```python
from build123d import *

# Parameters (mm, degrees)
SKETCH1_W              = 150
SKETCH1_H              = 150
BOSS_EXTRUDE1_DEPTH    = 25
SKETCH2_R              = 30
BOSS_EXTRUDE2_DEPTH    = 9
CHAMFER1_SIZE          = 2
M25X1_5_TAPPED_HOLE1_D = 23.5
HOLE1_D                = 17
HOLE1_CBORE_D          = 28
HOLE1_CBORE_DEPTH      = 15
CIRPATTERN1_COUNT      = 4


with BuildPart() as part:
    # Sketch1 → Boss-Extrude1 (new body)
    with BuildSketch(Plane(origin=(0, 0, 0), x_dir=(1, 0, 0), z_dir=(0, 1, 0))):
        Rectangle(SKETCH1_W, SKETCH1_H)
    extrude(amount=BOSS_EXTRUDE1_DEPTH)

    # Sketch2 → Boss-Extrude2 (add)
    with BuildSketch(Plane(origin=(0, 25, 0), x_dir=(1, 0, 0), z_dir=(0, 1, 0))):
        with Locations(Location((0, 0, 0), (0, 0, 270))):
            Circle(SKETCH2_R)
    extrude(amount=BOSS_EXTRUDE2_DEPTH)

    # Chamfer1
    chamfer1_edges = [part.edges().sort_by_distance(p)[0] for p in [
        (0, 34, -30),
    ]]
    chamfer(chamfer1_edges, length=CHAMFER1_SIZE)

    # M25x1.5 Tapped Hole1 (through all)
    with Locations(Plane(origin=(0, 34, 0), x_dir=(1, 0, 0), z_dir=(0, 1, 0))):
        with Locations((0, 0)):
            Hole(M25X1_5_TAPPED_HOLE1_D / 2)

    # Hole1 (through all)
    with Locations(Plane(origin=(0, 25, 0), x_dir=(1, 0, 0), z_dir=(0, 1, 0))):
        with Locations((-58, 58), (58, 58), (-58, -58), (58, -58)):
            CounterBoreHole(HOLE1_D / 2, HOLE1_CBORE_D / 2, HOLE1_CBORE_DEPTH)

    # Sketch7 → Cut-Revolve1 (revolve, cut)
    with BuildSketch(Plane.XY, mode=Mode.PRIVATE) as cut_revolve1_sk:
        Polygon((-65, 25), (-60, 20), (-60, 25), align=None)
    cut_revolve1 = revolve(cut_revolve1_sk.sketch.rotate(Axis((-60, 28.226297144, 0), (0, -1, 0)), 270), axis=Axis((-60, 28.226297144, 0), (0, -1, 0)), mode=Mode.SUBTRACT)

    # CirPattern1: Cut-Revolve1 ×4 about axis
    cirpattern1_axis = Axis((0, 0, 0), (0, 1, 0))
    for i in range(1, CIRPATTERN1_COUNT):
        add(cut_revolve1.rotate(cirpattern1_axis, i * 360 / CIRPATTERN1_COUNT), mode=Mode.SUBTRACT)


solid = part.part
```
Verification items for the finished model (mm, model axes). A direction names the side the tool comes from. Give positions to 0.01 mm unless a question says otherwise; leave off trailing zeros. Loops run counter-clockwise (first coordinate to the right, second up) from the corner with the lowest first, then second, coordinate; pieces in that order, holes last. Notation, with made-up numbers: M -9,-15 L 32,-15 A17 cw 32,-7 Z; hole C -3,32.5 d9. An arc over 180 degrees is marked long. Return JSON: item names as keys, results as strings.
1) Section check B-B, the plane z = 53. Enter the section's corners in (x, y), and give its area (3 significant figures).
Findings:
{"outline": "M -75,0 L -64.87,0 L -64.87,10 L -71.08,10 L -71.08,25 L -75,25 Z; M -51.13,0 L 51.13,0 L 51.13,10 L 44.92,10 L 44.92,25 L -44.92,25 L -44.92,10 L -51.13,10 Z; M 64.87,0 L 75,0 L 75,25 L 71.08,25 L 71.08,10 L 64.87,10 Z", "area": "2,690 mm2"}
2) Tool access check on faces 4 (the cylindrical face through (66.49, 4.93, 57.63)), 5 (the flat face through (-58, 10, -49)). Record the directions out of +Z, -Z, +X, -X, +Y, -Y that give a thin tool (end or side, any length) a straight path to the whole face; none if there is none.
Findings:
{"face 4": "+Y, -Y", "face 5": "+Y"}
3) Material ranges on L1, parallel to Z at x = -58, y = 8; L2, parallel to Z at x = -58, y = 18, recorded low to high. Write a range as [from, to].
Findings:
{"L1": "z = [-75, -66.5], [-49.5, 49.5], [66.5, 75]", "L2": "z = [-75, -72], [-44, 44], [72, 75]"}
4) Section check C-C, the plane x = -63. Count the separate pieces of the cut face and the enclosed holes in it, and give its area (3 significant figures).
Findings:
{"separate pieces": "3", "enclosed holes": "0", "area": "2,680 mm2"}
5) Mould release check, pull along Z, two halves, no side actions. Record for faces 1 (the flat face through (-1, 0, -18)), 2 (the flat face through (-1, 12, -75)), 3 (the conical face through (0, 21, 59)): released by +Z, released by -Z, zero draft, split by the parting line, or undercut.
Findings:
{"face 1": "zero draft", "face 2": "released by -Z", "face 3": "undercut"}
6) Gauge pin test, flat ends, axial feed: P1, Ø12, axis at x = -8, z = 5, coming from the +Y side; P2, Ø8.5, axis at x = 54.5, z = -63.5, coming from the +Y side; P3, Ø22.5, axis at x = -59, z = 53, coming from the +Y side. Record the tip position at first contact, or that the pin passes through.
Findings:
{"P1": "stops at y = 34", "P2": "stops at y = 10", "P3": "stops at y = 25"}
7) Section check A-A, the plane y = 13. Enter the section's corners in (x, z), and give its area (3 significant figures).
Findings:
{"outline": "M -75,-75 L 75,-75 L 75,75 L -75,75 Z; hole C -58,-58 d28; hole C -58,58 d28; hole C 0,0 d23.5; hole C 58,-58 d28; hole C 58,58 d28", "area": "19,600 mm2"}
